Read the model definition and answer for the solid it produces. Units are mm, in the model's axes. Face numbers are marked on the shaded views. A direction names the side the tool comes from. Give positions to 0.01 mm unless a question says otherwise; leave off trailing zeros. Order: outer loops, then holes, each group sorted by start corner. A loop starts at its lowest first (then second) coordinate and runs counter-clockwise, first axis right, second up. Notation, with made-up numbers: (-27, -19.75) - (17, -19.75) arc R7 ccw to (17, -11.75) - close; hole circle Ø10 at (-37, -26.5). An arc over 180 degrees is marked (long way). Return JSON: item names as keys, results as strings.
```python
from build123d import *

# Parameters (mm, degrees)
F1_DEPTH  = 39
F3_DEPTH  = 1
F5_DEPTH  = 1
F6_W      = 3
F6_H      = 41
F7_DEPTH  = 48
F8_W      = 4
F8_H      = 25
F9_DEPTH  = 30.001
F10_R     = 1.99999
F11_R     = 5
F12_W     = 15.2
F12_H     = 19.7
F13_DEPTH = 3
F15_DEPTH = 2
F17_DEPTH = 41
F19_DEPTH = 25
F21_DEPTH = 41


# Not quite as in the source:
# - a fillet or chamfer is up to 0.001 mm smaller than in the source, because OpenCascade refuses the exact size
# - ends of sketch curves that miss each other by under 0.0002 mm in the source are joined


with BuildPart() as f1:
    # F0 (on Top) → F1 (new body)
    with BuildSketch(Plane.XY):
        Polygon((0, -8), (0, 0), (-3, 0), (-3, -30), (23.763641715, -30), (23.763641715, -29), (-2, -29), (-2, -9), (0, -9), (4.8176753794, -21.2806219141), (5.7998719041, -21.4797707681), (19.5929166818, -24.2767604715), (27.2138139009, -27.8326366097), (28.2138139009, -27.8326366097), (28.2138139009, -25.9040332723), (28.2138139009, -25.0045752954), (6, -20.5), (6, -8), align=None)
    extrude(amount=F1_DEPTH)

    # F2 (on face) → F3 (join)
    with BuildSketch(Plane.XY.offset(39)):
        Polygon((0, 0), (-3, 0), (-3, -30), (23.763641715, -30), (28.2138139009, -27.8326366097), (28.2138139009, -25.0045752954), (6, -20.5), (6, -8), (0, -8), align=None)
    extrude(amount=F3_DEPTH)

    # F4 (on face) → F5 (join)
    with BuildSketch(Plane(origin=(0, 0, 0), x_dir=(1, 0, 0), z_dir=(0, 0, -1))):
        Polygon((-3, 0), (0, 0), (0, 8), (6, 8), (6, 20.5), (28.2138139009, 25.0045752954), (28.2138139009, 27.8326366097), (23.763641715, 30), (-3, 30), align=None)
    extrude(amount=F5_DEPTH)

    # F6 (on face) → F7 (join)
    with BuildSketch(Plane(origin=(-3, 0, 0), x_dir=(0, -1, 0), z_dir=(-1, 0, 0))):
        with Locations((28.5, 19.5)):
            Rectangle(F6_W, F6_H)
    extrude(amount=F7_DEPTH)

    # F8 (on face) → F9 (cut, through all)
    with BuildSketch(Plane.XZ.offset(30)):
        with Locations((-45.2, 19.5)):
            Rectangle(F8_W, F8_H)
    extrude(amount=-F9_DEPTH, mode=Mode.SUBTRACT)

    # F10 (radius 2 in the source; OpenCascade refuses exactly that, so slightly less here)
    f10_edges = [f1.edges().sort_by_distance(p)[0] for p in [
        (-47.2, -28.5, 32),
        (-43.2, -28.5, 32),
        (-47.2, -28.5, 7),
        (-43.2, -28.5, 7),
    ]]
    fillet(f10_edges, radius=F10_R)

    # F11
    f11_edges = [f1.edges().sort_by_distance(p)[0] for p in [
        (-51, -28.5, 40),
        (-51, -28.5, -1),
    ]]
    fillet(f11_edges, radius=F11_R)

    # F12 (on face) → F13 (cut)
    with BuildSketch(Plane(origin=(-3, 0, 0), x_dir=(0, -1, 0), z_dir=(-1, 0, 0))):
        with Locations((19.4, 19.5)):
            Rectangle(F12_W, F12_H)
    extrude(amount=-F13_DEPTH, mode=Mode.SUBTRACT)

    # F14 (on face) → F15 (join)
    with BuildSketch(Plane(origin=(-3, 0, 0), x_dir=(0, -1, 0), z_dir=(-1, 0, 0))):
        Polygon((10.8, 30.35), (10.8, 8.65), (27, 8.65), (27, 9.65), (11.8, 9.65), (11.8, 29.35), (27, 29.35), (27, 30.35), align=None)
    extrude(amount=-F15_DEPTH)

    # F16 (on face) → F17 (join, through all)
    with BuildSketch(Plane(origin=(0, 0, -1), x_dir=(1, 0, 0), z_dir=(0, 0, -1))):
        Polygon((-14, 0), (-3, 0), (-3, 8), (-14, 5.5), align=None)
    extrude(amount=-F17_DEPTH)

    # F18 (on face) → F19 (cut)
    with BuildSketch(Plane(origin=(-14, 0, 0), x_dir=(0, -1, 0), z_dir=(-1, 0, 0))):
        with BuildLine():
            Line((-0.9789119939, 3.5), (2.125, 3.5))
            ThreePointArc((2.125, 3.5), (4.25, 5.625), (2.125, 7.75))
            Line((2.125, 7.75), (-0.9789119939, 7.75))
            Line((-0.9789119939, 7.75), (-0.9789119939, 3.5))
        make_face()
        with BuildLine():
            Line((-0.98, 21.45), (2.125, 21.45))
            ThreePointArc((2.125, 21.45), (4.25, 23.575), (2.125, 25.7))
            Line((2.125, 25.7), (-0.98, 25.7))
            Line((-0.98, 25.7), (-0.98, 21.45))
        make_face()
    extrude(amount=-F19_DEPTH, mode=Mode.SUBTRACT)

    # F20 (on face) → F21 (join, through all)
    with BuildSketch(Plane.XY.offset(40)):
        Polygon((-3, -8), (-14, -5.5), (-3, -11.3482829183), align=None)
    extrude(amount=-F21_DEPTH)


solid = f1.part
```
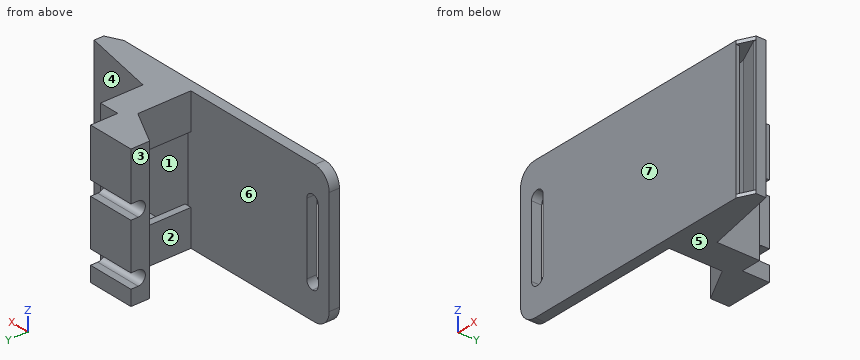
Q1. A cutting plane is placed at C-C (x = 17). Write down the section's boundary in (y, z), and give its area (3 significant figures).
Values:
{"outline": "(-30, -1) - (-22.73, -1) - (-22.73, 40) - (-30, 40) - close; hole (-29, 0) - (-23.75, 0) - (-23.75, 39) - (-29, 39) - close", "area": "93.3 mm²"}
Q2. A cutting plane is placed at D-D (y = -14). Write down the section's boundary in (x, z).
Values:
{"outline": "(-3, -1) - (6, -1) - (6, 40) - (-3, 40) - (-3, 29.35) - (-1, 29.35) - (-1, 30.35) - (-2, 30.35) - (-2, 39) - (1.96, 39) - (1.96, 0) - (-2, 0) - (-2, 8.65) - (-1, 8.65) - (-1, 9.65) - (-3, 9.65) - close"}
Q3. Determine the mould class of the marked faces 4, 5, 6 and 7 for opening direction Y: released by +Y, released by -Y, zero draft, split by the parting line, or undercut.
Values:
{"face 4": "released by +Y", "face 5": "zero draft", "face 6": "undercut", "face 7": "released by -Y"}
Q4. Consider L1, parallel to Z at x = 16, y = -24; L2, parallel to Y at x = -8, z = 15.5; L3, parallel to X at y = -19, z = 2. Determine where each line is inside the solid, lowest interval first.
Values:
{"L1": "z = -1 to 0, 39 to 40", "L2": "y = -30 to -27, -8.69 to 0", "L3": "x = -3 to -2, 3.92 to 6"}
Q5. For the marked faces 1, 2 and 3, determine the directions among +Z, -Z, +X, -X, +Y, -Y from which every point of the face is accessible in a straight line to the end or side of a thin tool.
Values:
{"face 1": "+X", "face 2": "+Z, -Z, -X", "face 3": "+Z, -Z, -X, +Y"}
Q6. Given pin 1 (12 mm diameter, centred on x = -25, z = 24.5, fed in from +Y); pin 2 (3 mm diameter, centred on y = -13, z = 20, fed in from -X); pin 3 (7.5 mm diameter, centred on x = 4.5, z = 20, fed in from +Y), each flat-ended and moving along its own axis, determine where each tip first touches the part or whether it passes through.
Values:
{"pin 1": "stops at y = -27", "pin 2": "stops at x = -3", "pin 3": "stops at y = -8"}
Q7. A cutting plane is placed at B-B (x = -7). Write down the section's boundary in (y, z) (3 decimals).
Values:
{"outline": "(-30, -1) - (-27, -1) - (-27, 40) - (-30, 40) - close; (-9.222, -1) - (0, -1) - (0, 3.5) - (-2.125, 3.5) arc R2.125 cw to (-2.125, 7.75) - (0, 7.75) - (0, 21.45) - (-2.125, 21.45) arc R2.125 cw to (-2.125, 25.7) - (0, 25.7) - (0, 40) - (-9.222, 40) - close"}
Q8. A cutting plane is placed at A-A (z = 16). Give the number of separate pieces and of enclosed holes in the cut face, and give its area (3 significant figures).
Values:
{"separate pieces": "3", "enclosed holes": "0", "area": "367 mm²"}
